The model under review builds one solid part; all positions refer to its coordinate system, in mm. Face numbers are marked on the shaded views. A direction names the side the tool comes from. Round coordinates to 2 decimals unless told otherwise and drop trailing zeros. Loops run counter-clockwise (first coordinate to the right, second up) from the corner with the lowest first, then second, coordinate; pieces in that order, holes last. Notation, with made-up numbers: M 42.25,67 L 65.25,67 A31 cw 65.25,98 Z; hole C 53.5,51 d11. An arc over 180 degrees is marked long. Return JSON: item names as keys, results as strings. Group by question number.
Q1. Consider section B-B (y = 0). State the section outline as (x, z) points, and give its area (3 significant figures).
Q2. Clearance check with flat-ended pins moving along their axes: pin 1 Ø6 at (x, y) = (107, -145) entering from +Z; pin 2 Ø1 at (x, y) = (-164.5, 144) entering from +Z; pin 3 Ø6 at (x, z) = (105, 37) entering from -Y. State where each tip first meets the part, or that it passes through.
Q3. Draft analysis for pull direction Y (two halves, no side actions). For the marked faces 1 and 2, state which applies: pulls with the +Y half, pulls with the -Y half, needs draft (parallel to the pull), parting line crosses it, or undercut.
Q4. For the marked faces 3 and 4, list the 3-axis set-ups (+Z, -Z, +X, -X, +Y, -Y) from which the entire face can be reached by the end or side of a thin tool; tool diameter is ignored.
Q5. To check wall thickness, follow line 1 along Z through (x, y) = (-34, -112.5); line 2 along X through (y, z) = (175, 244.5); line 3 along Z through (x, y) = (-171, -206.5). State the ranges of each line that lie inside material, in increasing order.
Q6. Consider section D-D (z = 126.5). State the section outline as (x, y) points.
Q7. Consider section A-A (x = 0). State the section outline as (y, z) points.
Q8. Consider section C-C (z = 157.5). State the section outline as (x, y) points.
from build123d import *

# Parameters (mm, degrees)
F3_DEPTH = 15


with BuildPart() as f1:
    # F0 (on Front) → F1 (revolve)
    with BuildSketch(Plane.XZ):
        Polygon((30, 55), (30, 15), (143.6414506771, 15), (150, 0), (162.4696655932, 0), (259.9674218774, 230), (268.4454876412, 250), (256.7487955093, 250), (256.7487955093, 257.3588024481), (238.7105971575, 257.3588024481), (238.7105971575, 250), (225, 250), (142.3388588025, 55), align=None)
        Polygon((268.4454876412, 250), (259.9674218774, 230), (278.4454876412, 230), (278.4454876412, 250), align=None)
    revolve(axis=Axis((0, 0, 38.856908679), (0, 0, 1)))

    # F2 (on face) → F3 (cut, through all)
    with BuildSketch(Plane(origin=(0, 0, 0), x_dir=(1, 0, 0), z_dir=(0, 0, -1))):
        with BuildLine():
            Line((-62.1744492844, 150.1023986955), (-57.4025148548, 138.5819298767))
            ThreePointArc((-57.4025148548, 138.5819298767), (0, 150), (57.4025148548, 138.5819298767))
            Line((57.4025148548, 138.5819298767), (62.1744492844, 150.1023986955))
            ThreePointArc((62.1744492844, 150.1023986955), (0, 162.4696655932), (-62.1744492844, 150.1023986955))
        make_face()
        with BuildLine():
            ThreePointArc((148.7167292061, -19.578928833), (129.9038105677, -75), (91.3142143513, -119.0030010437))
            Line((91.3142143513, -119.0030010437), (98.9052657971, -128.8958518943))
            ThreePointArc((98.9052657971, -128.8958518943), (140.702857748, -81.2348327966), (161.0797150815, -21.2065468011))
            Line((161.0797150815, -21.2065468011), (148.7167292061, -19.578928833))
        make_face()
        with BuildLine():
            ThreePointArc((-91.3142143513, -119.0030010437), (-129.9038105677, -75), (-148.7167292061, -19.578928833))
            Line((-148.7167292061, -19.578928833), (-161.0797150815, -21.2065468011))
            ThreePointArc((-161.0797150815, -21.2065468011), (-140.702857748, -81.2348327966), (-98.9052657971, -128.8958518943))
            Line((-98.9052657971, -128.8958518943), (-91.3142143513, -119.0030010437))
        make_face()
        with BuildLine():
            Line((-91.3142143513, -119.0030010437), (0, 0))
            Line((0, 0), (-148.7167292061, -19.578928833))
            ThreePointArc((-148.7167292061, -19.578928833), (-129.9038105677, -75), (-91.3142143513, -119.0030010437))
        make_face()
        with BuildLine():
            Line((-57.4025148548, 138.5819298767), (0, 0))
            Line((0, 0), (57.4025148548, 138.5819298767))
            ThreePointArc((57.4025148548, 138.5819298767), (0, 150), (-57.4025148548, 138.5819298767))
        make_face()
        with BuildLine():
            Line((148.7167292061, -19.578928833), (0, 0))
            Line((0, 0), (91.3142143513, -119.0030010437))
            ThreePointArc((91.3142143513, -119.0030010437), (129.9038105677, -75), (148.7167292061, -19.578928833))
        make_face()
        with BuildLine():
            Line((-82.5295173068, 199.2438799781), (-62.1744492844, 150.1023986955))
            ThreePointArc((-62.1744492844, 150.1023986955), (0, 162.4696655932), (62.1744492844, 150.1023986955))
            Line((62.1744492844, 150.1023986955), (82.5295173068, 199.2438799781))
            Line((82.5295173068, 199.2438799781), (-82.5295173068, 199.2438799781))
        make_face()
        with BuildLine():
            ThreePointArc((-98.9052657971, -128.8958518943), (-140.702857748, -81.2348327966), (-161.0797150815, -21.2065468011))
            Line((-161.0797150815, -21.2065468011), (-213.815020263, -28.1492814393))
            Line((-213.815020263, -28.1492814393), (-131.2855029562, -171.0945985388))
            Line((-131.2855029562, -171.0945985388), (-98.9052657971, -128.8958518943))
        make_face()
        with BuildLine():
            ThreePointArc((161.0797150815, -21.2065468011), (140.702857748, -81.2348327966), (98.9052657971, -128.8958518943))
            Line((98.9052657971, -128.8958518943), (131.2855029562, -171.0945985388))
            Line((131.2855029562, -171.0945985388), (213.815020263, -28.1492814393))
            Line((213.815020263, -28.1492814393), (161.0797150815, -21.2065468011))
        make_face()
    extrude(amount=-F3_DEPTH, mode=Mode.SUBTRACT)


solid = f1.part
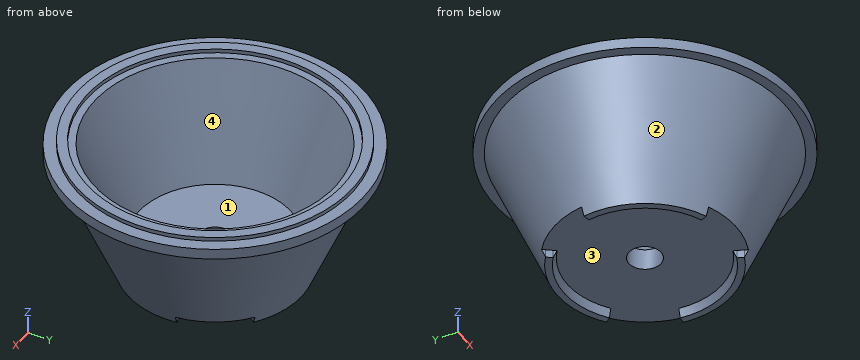
Values:
{
 "1": {"outline": "M -278.45,230 L -259.97,230 L -162.47,0 L -150,0 L -143.64,15 L -30,15 L -30,55 L -142.34,55 L -225,250 L -238.71,250 L -238.71,257.36 L -256.75,257.36 L -256.75,250 L -278.45,250 Z; M 30,15 L 143.64,15 L 150,0 L 162.47,0 L 259.97,230 L 278.45,230 L 278.45,250 L 256.75,250 L 256.75,257.36 L 238.71,257.36 L 238.71,250 L 225,250 L 142.34,55 L 30,55 Z", "area": "30,100 mm2"},
 "2": {"pin 1": "stops at z = 151.41", "pin 2": "stops at z = 236.14", "pin 3": "stops at y = -146.58"},
 "3": {"face 1": "undercut", "face 2": "parting line crosses it"},
 "4": {"face 3": "-Z", "face 4": "+Z"},
 "5": {"line 1": "z = 15 to 55", "line 2": "x = -216.58 to -137.68, 137.68 to 216.58", "line 3": "z = 230 to 250"},
 "6": {"outline": "C 0,0 d432.19; hole C 0,0 d345.3"},
 "7": {"outline": "M -278.45,230 L -259.97,230 L -168.83,15 L -30,15 L -30,55 L -142.34,55 L -225,250 L -238.71,250 L -238.71,257.36 L -256.75,257.36 L -256.75,250 L -278.45,250 Z; M 30,15 L 143.64,15 L 150,0 L 162.47,0 L 259.97,230 L 278.45,230 L 278.45,250 L 256.75,250 L 256.75,257.36 L 238.71,257.36 L 238.71,250 L 225,250 L 142.34,55 L 30,55 Z"},
 "8": {"outline": "C 0,0 d458.47; hole C 0,0 d371.58"}
}
